```python
from build123d import *

# Parameters (mm, degrees)
BOSS_EXTRUDE1_DEPTH = 15.5
CHAMFER1_START      = 3
CHAMFER1_DEPTH      = 16
CIRPATTERN1_COUNT   = 3
SKETCH4_R           = 1.75
CUT_EXTRUDE1_DEPTH  = 12
CIRPATTERN2_COUNT   = 3
SKETCH5_R           = 1.75
CUT_EXTRUDE2_DEPTH  = 43.852946223
CIRPATTERN3_COUNT   = 3


with BuildPart() as part:
    # Sketch2 → Revolve1 (revolve)
    with BuildSketch(Plane(origin=(0, 0, 0), x_dir=(0, 0, -1), z_dir=(1, 0, 0)), mode=Mode.PRIVATE) as revolve1_sk:
        Polygon((0, 28.25), (-3, 28.25), (-3, 18.5), (0, 18.5), (2, 18.5), (2, 28.25), align=None)
    revolve(revolve1_sk.sketch.rotate(Axis((0, 0, 0), (0, 0, 1)), 90), axis=Axis((0, 0, 0), (0, 0, 1)))

    # Sketch3 → Boss-Extrude1 (add)
    with BuildSketch(Plane.XY.offset(3)):
        with BuildLine():
            Line((-7.524627897, 16.900590966), (-11.490310167, 25.807659178))
            ThreePointArc((-11.490310167, 25.807659178), (0, 28.25), (11.490310167, 25.807659178))
            Line((11.490310167, 25.807659178), (7.524627897, 16.900590966))
            ThreePointArc((7.524627897, 16.900590966), (0, 18.5), (-7.524627897, 16.900590966))
        make_face()
    boss_extrude1 = extrude(amount=BOSS_EXTRUDE1_DEPTH)

    # Chamfer1: read off the stored shape, not the designer's step
    # Chamfer1 outline → Chamfer1 (cut)
    with BuildSketch(Plane.XY.offset(CHAMFER1_START)):
        with BuildLine():
            Line((7.524627897, 16.900590966), (9.558311113, 21.468318255))
            Line((9.558311113, 21.468318255), (5.263960206, 17.735295964))
            ThreePointArc((5.263960206, 17.735295964), (6.407899775, 17.354792435), (7.524627897, 16.900590966))
        make_face()
        with BuildLine():
            ThreePointArc((-7.524627897, 16.900590966), (-6.407899775, 17.354792435), (-5.263960206, 17.735295964))
            Line((-5.263960206, 17.735295964), (-9.558311112, 21.468318255))
            Line((-9.558311112, 21.468318255), (-7.524627897, 16.900590966))
        make_face()
    chamfer1 = extrude(amount=CHAMFER1_DEPTH, mode=Mode.SUBTRACT)

    # CirPattern1: Boss-Extrude1, Chamfer1 ×3 about axis
    cirpattern1_axis = Axis((0, 0, 0), (0, 0, 1))
    add([boss_extrude1.rotate(cirpattern1_axis, i * 360 / CIRPATTERN1_COUNT) for i in range(1, CIRPATTERN1_COUNT)])
    add([chamfer1.rotate(cirpattern1_axis, i * 360 / CIRPATTERN1_COUNT) for i in range(1, CIRPATTERN1_COUNT)], mode=Mode.SUBTRACT)

    # Sketch4 → Cut-Extrude1 (cut)
    with BuildSketch(Plane.XY.offset(18.5)):
        with Locations((0, 23.25)):
            Circle(SKETCH4_R)
    cut_extrude1 = extrude(amount=-CUT_EXTRUDE1_DEPTH, mode=Mode.SUBTRACT)

    # CirPattern2: Cut-Extrude1 ×3 about axis
    cirpattern2_axis = Axis((0, 0, 0), (0, 0, 1))
    for i in range(1, CIRPATTERN2_COUNT):
        add(cut_extrude1.rotate(cirpattern2_axis, i * 360 / CIRPATTERN2_COUNT), mode=Mode.SUBTRACT)

    # Sketch5 → Cut-Extrude2 (cut, through all)
    with BuildSketch(Plane.XY.offset(3)):
        with Locations((0, -23.25)):
            Circle(SKETCH5_R)
    cut_extrude2 = extrude(amount=-CUT_EXTRUDE2_DEPTH, mode=Mode.SUBTRACT)

    # CirPattern3: Cut-Extrude2 ×3 about axis
    cirpattern3_axis = Axis((0, 0, 0), (0, 0, 1))
    for i in range(1, CIRPATTERN3_COUNT):
        add(cut_extrude2.rotate(cirpattern3_axis, i * 360 / CIRPATTERN3_COUNT), mode=Mode.SUBTRACT)


solid = part.part
```
Geometry: final body of the model. Coordinates: model frame, mm. A direction names the side the tool comes from. Round coordinates to 2 decimals unless told otherwise and drop trailing zeros. Order: outer loops, then holes, each group sorted by start corner. A loop starts at its lowest first (then second) coordinate and runs counter-clockwise, first axis right, second up. Notation, with made-up numbers: (15.25, 70.5) -> (37.25, 70.5) arc R24 ccw to (37.25, 84.5) -> close; hole circle Ø1 at (43.5, 51). An arc over 180 degrees is marked (long way). Write each question's results on one line, items separated by ' | '.
Q1. Section query C-C (z = 4.25). Output: boundary loops of the cut face in (x, y), and give its area (3 significant figures).
Response values:
outline: (-28.1, -2.95) arc R28.25 ccw to (-16.6, -22.85) -> (-13.81, -19.01) -> (-12.73, -13.43) arc R18.5 cw to (-17.99, -4.31) -> (-23.37, -2.46) -> close; (-11.49, 25.81) -> (-9.56, 21.47) -> (-5.26, 17.74) arc R18.5 cw to (5.26, 17.74) -> (9.56, 21.47) -> (11.49, 25.81) arc R28.25 ccw to start; (12.73, -13.43) -> (13.81, -19.01) -> (16.6, -22.85) arc R28.25 ccw to (28.1, -2.95) -> (23.37, -2.46) -> (17.99, -4.31) arc R18.5 cw to start | area: 537 mm²
Q2. Section query D-D (z = 7.5). Output: boundary loops of the cut face in (x, y) (3 decimals), and give its area (3 significant figures).
Response values:
outline: (-28.095, -2.953) arc R28.25 ccw to (-16.605, -22.855) -> (-13.813, -19.012) -> (-12.727, -13.426) arc R18.5 cw to (-17.991, -4.309) -> (-23.371, -2.456) -> close; (-11.49, 25.808) -> (-9.558, 21.468) -> (-5.264, 17.735) arc R18.5 cw to (5.264, 17.735) -> (9.558, 21.468) -> (11.49, 25.808) arc R28.25 ccw to start; (12.727, -13.426) -> (13.813, -19.012) -> (16.605, -22.855) arc R28.25 ccw to (28.095, -2.953) -> (23.371, -2.456) -> (17.991, -4.309) arc R18.5 cw to start; hole circle Ø3.5 at (-20.135, -11.625); hole circle Ø3.5 at (0, 23.25); hole circle Ø3.5 at (20.135, -11.625) | area: 508 mm²
Q3. Ray query, line 1 along Z through (x, y) = (-18.5, 3); line 2 along X through (y, z) = (-18, 14); line 3 along X through (y, z) = (-6.5, 16.5). Return the intervals inside material, ascending.
Response values:
line 1: -2 to 3 | line 2: -21.77 to -13.62, 13.62 to 21.77 | line 3: -27.49 to -17.32, 17.32 to 27.49
Q4. Access query for faces 1 (the face through (20, -12, 6.5)), 2 (the face through (13.28, -16.26, 10.64)), 3 (the face through (7.441, 19.628, 10.642)). Directions: +Z, -Z, +X, -X, +Y, -Y. A direction counts if a zero-diameter tool reaches every point of the face in a straight line with its end or side. Return the directions, or none.
Response values:
face 1: +Z | face 2: +Z, -Y | face 3: +Z, +X, -Y
Q5. Section query A-A (y = 0). Output: boundary loops of the cut face in (x, z), and give its area (3 significant figures).
Response values:
outline: (-28.25, -2) -> (-18.5, -2) -> (-18.5, 3) -> (-28.25, 3) -> close; (18.5, -2) -> (28.25, -2) -> (28.25, 3) -> (18.5, 3) -> close | area: 97.5 mm²
Q6. Pin query (flat end, axial travel): pin 1 Ø1 at (x, y) = (19.5, -11.5) entering from +Z; pin 2 Ø6 at (x, z) = (1.5, 2.5) entering from +Y; pin 3 Ø1 at (y, z) = (-0.5, 11.5) entering from -X; pin 4 Ø10 at (y, z) = (-4.5, 5) entering from +X. Return the tip coordinate at first contact, or that it passes through.
Response values:
pin 1: z = 6.5 | pin 2: y = 28.25 | pin 3: through | pin 4: x = 28.25
Q7. Section query B-B (x = 0). Output: boundary loops of the cut face in (y, z), and give its area (3 significant figures).
Response values:
outline: (-28.25, -2) -> (-25, -2) -> (-25, 3) -> (-28.25, 3) -> close; (-21.5, -2) -> (-18.5, -2) -> (-18.5, 3) -> (-21.5, 3) -> close; (18.5, -2) -> (28.25, -2) -> (28.25, 18.5) -> (25, 18.5) -> (25, 6.5) -> (21.5, 6.5) -> (21.5, 18.5) -> (18.5, 18.5) -> close | area: 189 mm²
